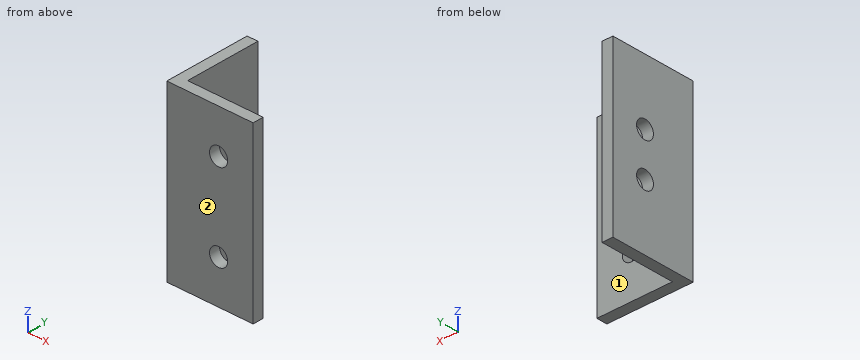
from build123d import *

# Parameters (mm, degrees)
SKETCH2_W           = 22.225
SKETCH2_H           = 3.175
SKETCH2_W_2         = 3.175
SKETCH2_H_2         = 22.225
BOSS_EXTRUDE1_DEPTH = 50.8
SKETCH3_R           = 2.667
CUT_EXTRUDE1_DEPTH  = 3.175
SKETCH4_R           = 2.667
CUT_EXTRUDE2_DEPTH  = 3.175


with BuildPart() as part:
    # Sketch2 → Boss-Extrude1 (new body)
    with BuildSketch(Plane.XY):
        with Locations((14.2875, 1.5875)):
            Rectangle(SKETCH2_W, SKETCH2_H)
        with Locations((1.5875, 1.5875)):
            Rectangle(SKETCH2_W_2, SKETCH2_H)
        with Locations((1.5875, 14.2875)):
            Rectangle(SKETCH2_W_2, SKETCH2_H_2)
    extrude(amount=BOSS_EXTRUDE1_DEPTH)

    # Sketch3 → Cut-Extrude1 (cut)
    with BuildSketch(Plane.ZY):
        with Locations((19.05, 15.24)):
            Circle(SKETCH3_R)
        with Locations((31.75, 15.24)):
            Circle(SKETCH3_R)
    extrude(amount=-CUT_EXTRUDE1_DEPTH, mode=Mode.SUBTRACT)

    # Sketch4 → Cut-Extrude2 (cut)
    with BuildSketch(Plane.XZ):
        with Locations((15.24, 38.1)):
            Circle(SKETCH4_R)
        with Locations((15.24, 12.7)):
            Circle(SKETCH4_R)
    extrude(amount=-CUT_EXTRUDE2_DEPTH, mode=Mode.SUBTRACT)


solid = part.part
Geometry check sheet. Reference: the model listing, model coordinates, mm. Face numbers are marked on the shaded views. A direction names the side the tool comes from. Round coordinates to 2 decimals unless told otherwise and drop trailing zeros. Write each loop counter-clockwise with the first axis right and the second up, starting at its lowest first coordinate (ties: lowest second). Pieces come first, ordered by that corner, then holes.
Item 1: Section check A-A (y = 15.24). Record the boundary of the cut face in (x, z) (3 decimals).
Determined:
outline: (0, 0) - (3.175, 0) - (3.175, 16.383) - (0, 16.383) - close; (0, 21.717) - (3.175, 21.717) - (3.175, 29.083) - (0, 29.083) - close; (0, 34.417) - (3.175, 34.417) - (3.175, 50.8) - (0, 50.8) - close
Item 2: Go/stop test with flat-tipped pins: pin 1 Ø3 at (y, z) = (8.5, 29.5) entering from -X; pin 2 Ø3 at (x, y) = (17, 5) entering from -Z; pin 3 Ø7 at (x, z) = (15.24, 12.7) entering from +Y (3 decimals); pin 4 Ø11 at (y, z) = (16.5, 24.5) entering from +X (3 decimals). Record where each tip stops, or that it passes through.
Determined:
pin 1: stops at x = 0
pin 2: passes through
pin 3: stops at y = 3.175
pin 4: stops at x = 3.175
Item 3: Material ranges on line 1 along Z through (x, y) = (15.24, 2.4); line 2 along Y through (x, z) = (10.5, 16) (3 decimals), recorded low to high.
Determined:
line 1: z = 0 to 10.03, 15.37 to 35.43, 40.77 to 50.8
line 2: y = 0 to 3.175
Item 4: Access from +Z, -Z, +X, -X, +Y, -Y to the whole of each face (thin tool, end or side, straight path). Record for the marked faces 1 and 2.
Determined:
face 1: +Z, -Z, +X, +Y
face 2: +Z, -Z, +X, -X, -Y
Item 5: Section check D-D (z = 26). Record the boundary of the cut face in (x, y) (3 decimals), plus the area to 3 significant figures.
Determined:
outline: (0, 0) - (25.4, 0) - (25.4, 3.175) - (3.175, 3.175) - (3.175, 25.4) - (0, 25.4) - close
area: 151 mm2
Item 6: Section check B-B (z = 31.75). Record the boundary of the cut face in (x, y) (3 decimals), plus the area to 3 significant figures.
Determined:
outline: (0, 0) - (25.4, 0) - (25.4, 3.175) - (3.175, 3.175) - (3.175, 12.573) - (0, 12.573) - close; (0, 17.907) - (3.175, 17.907) - (3.175, 25.4) - (0, 25.4) - close
area: 134 mm2
Item 7: Section check C-C (x = 15.24). Record the boundary of the cut face in (y, z) (3 decimals).
Determined:
outline: (0, 0) - (3.175, 0) - (3.175, 10.033) - (0, 10.033) - close; (0, 15.367) - (3.175, 15.367) - (3.175, 35.433) - (0, 35.433) - close; (0, 40.767) - (3.175, 40.767) - (3.175, 50.8) - (0, 50.8) - close
